```python
from build123d import *

# Parameters (mm, degrees)
PAD003_DEPTH = 3.5
POCKET_DEPTH = 5.5


with BuildPart() as obj1:
    # Sketch010 → Pad003 (new body, symmetric)
    with BuildSketch(Plane.XY):
        with BuildLine():
            ThreePointArc((59.498979, 20.271308), (30.157918, 27.585958), (0, 29.8))
            Line((0, 29.8), (0, 16.6))
            ThreePointArc((58.317055, 0.623642), (30.232941, 12.533656), (0, 16.6))
            ThreePointArc((58.317055, 0.623642), (63.354776, 0.781276), (65.351677, 5.409004))
            Line((63.7883, 15.177117), (65.351677, 5.409004))
            ThreePointArc((63.7883, 15.177117), (62.350118, 18.319069), (59.498979, 20.271308))
        make_face()
    extrude(amount=PAD003_DEPTH, both=True)

    # Sketch009 → Pocket (cut)
    with BuildSketch(Plane.XY.offset(3.5)):
        with BuildLine():
            Line((0, 27.898268), (0, 18.183007))
            ThreePointArc((57.375322, 3.010124), (29.674349, 14.327664), (0, 18.183007))
            ThreePointArc((57.375322, 3.010124), (58.546948, 3.277627), (58.382807, 4.46814))
            ThreePointArc((58.112759, 15.405314), (55.75963, 9.875292), (58.382807, 4.46814))
            ThreePointArc((58.112759, 15.405314), (58.750082, 17.397997), (57.35497, 18.957045))
            ThreePointArc((57.35497, 18.957045), (29.050369, 25.819583), (0, 27.898268))
        make_face()
    extrude(amount=-POCKET_DEPTH, mode=Mode.SUBTRACT)

    # Sketch011 (on Face2 of Pocket) → Groove (revolve, cut)
    with BuildSketch(Plane(origin=(62.588677, 10.017255, 0), x_dir=(-0.158038, 0.987433, 0), z_dir=(0.987433, 0.158038, 0))):
        with BuildLine():
            Line((0, -3.6), (0, 3.6))
            Line((0, 3.6), (5, 3.6))
            ThreePointArc((5, 3.6), (4.4, 3), (5, 2.4))
            Line((5, -2.4), (5, 2.4))
            ThreePointArc((5, -2.4), (4.400007, -3), (5, -3.6))
            Line((0, -3.6), (5, -3.6))
        make_face()
    revolve(axis=Axis((62.588677, 10.017255, 0), (0, 0, 1)), mode=Mode.SUBTRACT)


with BuildPart() as part_mirroring:
    # Part__Mirroring: instance of obj1
    add(obj1.part.mirror(Plane(origin=(0, 0, 0), x_dir=(0, -1, 0), z_dir=(1, 0, 0))))


solid = part_mirroring.part
```
Can you work these out from the model? Positions are in its coordinate system, mm. A direction names the side the tool comes from. Give positions to 0.01 mm unless a question says otherwise; leave off trailing zeros. Loops run counter-clockwise (first coordinate to the right, second up) from the corner with the lowest first, then second, coordinate; pieces in that order, holes last. Notation, with made-up numbers: M 17.25,60.5 L 40.25,60.5 A7 cw 40.25,64.5 Z; hole C 54,-5.75 d7. An arc over 180 degrees is marked long. One line per question, with ' | ' between items. Start each with the question number.
Q1. If we section it at C-C (y = 24): Please give me the cut outline in (x, z), plus the area to 3 significant figures.
Q2. If we section it at D-D (x = -13): Please give me the cut outline in (y, z), plus the area to 3 significant figures.
Q3. If we mould it in two halves opening along Y, with no side actions, what happens to faces 4 (the cylindrical face through (-29.454, 25.756, 0.788)), 5 (the cylindrical face through (-58.536, 3.263, 0.788)), 6 (the cylindrical face through (-62.382, 18.281, 0.049)), 7 (the cylindrical face through (-30.65, 12.42, 0.05))? For each: +Y half, -Y half, draft (parallel to the pull), parting line (faces both ways), or undercut.
Q4. If I drill on line 1 (Y direction, x = -58, z = 0); line 2 (Z direction, x = -30.5, y = 22.25); line 3 (Y direction, x = -37, z = 1.25), over which ranges is the centre line in solid material (lowest first)? Write a range as from..to.
Q5. If we section it at A-A (x = -35): Please give me the cut outline in (y, z).
Q6. For faces 1 (the flat face through (0, 23.3, -2.3)), 2 (the flat face through (-29, 18, -2)), 3 (the cylindrical face through (-57.631, 9.364, 0.034)), which set-ups out of +Z, -Z, +X, -X, +Y, -Y let a thin tool reach every point of the face, with its end or its side?
Q7. For pin 1 Ø3 at (x, z) = (-50, -1) entering from -Y; pin 2 Ø1.5 at (x, z) = (-33.5, 1) entering from -Y; pin 3 Ø4 at (x, z) = (-23, -2.5) entering from -Y, each with a flat end and sliding along its axis, tell me the tip position at first contact or that it passes through.
Q8. If we section it at B-B (z = 0.75): Please give me the cut outline in (x, y).
Computed:
1) outline: M -47.16,-3.5 L 0,-3.5 L 0,-2 L -38.87,-2 L -38.87,3.5 L -47.16,3.5 Z | area: 116 mm²
2) outline: M 15.86,-3.5 L 29.48,-3.5 L 29.48,3.5 L 27.57,3.5 L 27.57,-2 L 17.45,-2 L 17.45,3.5 L 15.86,3.5 Z | area: 39.7 mm²
3) face 4: undercut | face 5: undercut | face 6: +Y half | face 7: -Y half
4) line 1: y = 0.81..2.91, 4.81..8.03, 12..15.3, 18.61..20.78 | line 2: z = -3.5..-2 | line 3: y = 10.45..12.13, 24.39..26.35
5) outline: M 11.12,-3.5 L 26.74,-3.5 L 26.74,3.5 L 24.79,3.5 L 24.79,-2 L 12.78,-2 L 12.78,3.5 L 11.12,3.5 Z
6) face 1: +Z, -Z, +X, +Y, -Y | face 2: +Z | face 3: none
7) pin 1: stops at y = 4.36 | pin 2: stops at y = 11.35 | pin 3: stops at y = 13.84
8) outline: M -65.35,5.41 A4.7 ccw -58.32,0.62 A114.42 cw 0,16.6 L 0,18.18 A116.01 ccw -57.38,3.01 A0.89 cw -58.38,4.47 A7.26 ccw -58.11,15.41 A2.11 cw -57.35,18.96 A175.2 cw 0,27.9 L 0,29.8 A177.02 ccw -59.5,20.27 A6.46 ccw -63.79,15.18 L -63.84,14.86 A5 cw long -65.29,5.81 Z
